Input: part model. Units: mm. Frame: model coordinates. A direction names the side the tool comes from. Give positions to 0.01 mm unless a question says otherwise; leave off trailing zeros. Loops run counter-clockwise (first coordinate to the right, second up) from the corner with the lowest first, then second, coordinate; pieces in that order, holes last. Notation, with made-up numbers: (61.5, 44) -> (73.5, 44) arc R17 ccw to (73.5, 64) -> close; hole circle Ø8 at (50, 2). An arc over 180 degrees is marked (long way). Answer as a JSON object with one key per item and string values.
```python
from build123d import *

# Parameters (mm, degrees)
CROQUIS1_W              = 25
CROQUIS1_H              = 25
CROQUIS1_W_2            = 22.6
CROQUIS1_H_2            = 22.6
SALIENTE_EXTRUIR1_DEPTH = 190
CROQUIS2_R              = 2.5
CORTAR_EXTRUIR1_DEPTH   = 193.044916621
CROQUIS3_R              = 40
CORTAR_EXTRUIR2_DEPTH   = 86


with BuildPart() as part:
    # Croquis1 → Saliente-Extruir1 (new body)
    with BuildSketch(Plane.XY):
        Rectangle(CROQUIS1_W, CROQUIS1_H)
        Rectangle(CROQUIS1_W_2, CROQUIS1_H_2, mode=Mode.SUBTRACT)
    extrude(amount=SALIENTE_EXTRUIR1_DEPTH)

    # Croquis2 → Cortar-Extruir1 (cut, through all)
    with BuildSketch(Plane(origin=(12.5, 0, 0), x_dir=(0, 0, -1), z_dir=(1, 0, 0))):
        with Locations(Location((-7, 0, 0), (0, 0, 90))):
            Circle(CROQUIS2_R)
        with Locations(Location((-183, 0, 0), (0, 0, 90))):
            Circle(CROQUIS2_R)
    extrude(amount=-CORTAR_EXTRUIR1_DEPTH, mode=Mode.SUBTRACT)

    # Croquis3 → Cortar-Extruir2 (cut)
    with BuildSketch(Plane(origin=(0, 0, 0), x_dir=(-1, 0, 0), z_dir=(0, 0, -1))):
        Circle(CROQUIS3_R)
        with BuildLine():
            Line((-11.5, 12.5), (11.5, 12.5))
            ThreePointArc((11.5, 12.5), (12.207106781, 12.207106781), (12.5, 11.5))
            Line((12.5, 11.5), (12.5, -11.5))
            ThreePointArc((12.5, -11.5), (12.207106781, -12.207106781), (11.5, -12.5))
            Line((11.5, -12.5), (-11.5, -12.5))
            ThreePointArc((-11.5, -12.5), (-12.207106781, -12.207106781), (-12.5, -11.5))
            Line((-12.5, -11.5), (-12.5, 11.5))
            ThreePointArc((-12.5, 11.5), (-12.207106781, 12.207106781), (-11.5, 12.5))
        make_face(mode=Mode.SUBTRACT)
    extrude(amount=-CORTAR_EXTRUIR2_DEPTH, mode=Mode.SUBTRACT)


solid = part.part
```
Q1. Section B-B, the plane z = 7. Return the cut outline in (x, y), then the cut area to 3 significant figures.
Evaluation:
{"outline": "(-12.5, -11.5) arc R1 ccw to (-11.5, -12.5) -> (11.5, -12.5) arc R1 ccw to (12.5, -11.5) -> (12.5, -2.5) -> (11.3, -2.5) -> (11.3, -11.3) -> (-11.3, -11.3) -> (-11.3, -2.5) -> (-12.5, -2.5) -> close; (-12.5, 2.5) -> (-11.3, 2.5) -> (-11.3, 11.3) -> (11.3, 11.3) -> (11.3, 2.5) -> (12.5, 2.5) -> (12.5, 11.5) arc R1 ccw to (11.5, 12.5) -> (-11.5, 12.5) arc R1 ccw to (-12.5, 11.5) -> close", "area": "101 mm2"}
Q2. Section D-D, the plane z = 135.5. Return the cut outline in (x, y), then the cut area to 3 significant figures.
Evaluation:
{"outline": "(-12.5, -12.5) -> (12.5, -12.5) -> (12.5, 12.5) -> (-12.5, 12.5) -> close; hole (-11.3, -11.3) -> (11.3, -11.3) -> (11.3, 11.3) -> (-11.3, 11.3) -> close", "area": "114 mm2"}
Q3. Draft query along Y for faces 1 (the flat face through (0, -12.5, 94)), 2 (the cylindrical face through (-11.89, -0.33, 185.48)), 3 (the flat face through (12.5, 0, 94)). Return one class per face: +Y half, -Y half, draft (parallel to the pull), parting line (faces both ways), or undercut.
Evaluation:
{"face 1": "-Y half", "face 2": "undercut", "face 3": "draft"}
Q4. Section A-A, the plane y = -5.25. Return the cut outline in (x, z), then the cut area to 3 significant figures.
Evaluation:
{"outline": "(-12.5, 0) -> (-11.3, 0) -> (-11.3, 190) -> (-12.5, 190) -> close; (11.3, 0) -> (12.5, 0) -> (12.5, 190) -> (11.3, 190) -> close", "area": "456 mm2"}
Q5. Ray query, line 1 along Z through (x, y) = (-11.55, 0); line 2 along Y through (x, z) = (1, 58). Return the intervals inside material, ascending.
Evaluation:
{"line 1": "z = 0 to 4.5, 9.5 to 180.5, 185.5 to 190", "line 2": "y = -12.5 to -11.3, 11.3 to 12.5"}
Q6. Access query for faces 4 (the flat face through (0, -11.3, 94)), 5 (the cylindrical face through (11.91, -0.33, 185.48)). Directions: +Z, -Z, +X, -X, +Y, -Y. A direction counts if a zero-diameter tool reaches every point of the face in a straight line with its end or side. Return the directions, or none.
Evaluation:
{"face 4": "+Z, -Z", "face 5": "+X, -X"}
